Check sheet for the modelled part. Datum: model origin and axes. Units: mm. Give positions to 0.01 mm unless a question says otherwise; leave off trailing zeros. Loops run counter-clockwise (first coordinate to the right, second up) from the corner with the lowest first, then second, coordinate; pieces in that order, holes last. Notation, with made-up numbers: (57, 34.25) - (75, 34.25) arc R19 cw to (75, 63.25) - close; hole circle Ø1 at (65.5, -18). An arc over 180 degrees is marked (long way). Use CSV: the item, a comma, the result in double quotes.
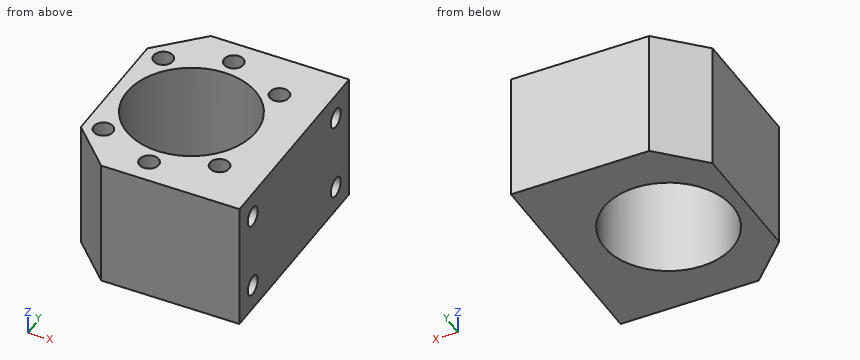
from build123d import *

# Parameters (mm, degrees)
SKETCH1_R           = 20
BOSS_EXTRUDE2_DEPTH = 40
SKETCH8_R           = 3
CUT_EXTRUDE1_DEPTH  = 16
SKETCH9_R           = 3
CUT_EXTRUDE2_DEPTH  = 16


with BuildPart() as part:
    # Sketch1 → Boss-Extrude2 (new body)
    with BuildSketch(Plane.XY):
        Polygon((-24, -20), (-11, -33), (31.93, -33), (31.93, 33), (-11, 33), (-24, 20), align=None)
        Circle(SKETCH1_R, mode=Mode.SUBTRACT)
    extrude(amount=BOSS_EXTRUDE2_DEPTH)

    # Sketch8 → Cut-Extrude1 (cut)
    with BuildSketch(Plane.XY.offset(40)):
        with Locations((0, 25.5)):
            Circle(SKETCH8_R)
        with Locations((18.03122292, 18.03122292)):
            Circle(SKETCH8_R)
        with Locations((18.03122292, -18.03122292)):
            Circle(SKETCH8_R)
        with Locations((0, -25.5)):
            Circle(SKETCH8_R)
        with Locations((-18.03122292, -18.03122292)):
            Circle(SKETCH8_R)
        with Locations((-18.03122292, 18.03122292)):
            Circle(SKETCH8_R)
    extrude(amount=-CUT_EXTRUDE1_DEPTH, mode=Mode.SUBTRACT)

    # Sketch9 → Cut-Extrude2 (cut)
    with BuildSketch(Plane(origin=(31.93, 0, 0), x_dir=(0, 0, -1), z_dir=(1, 0, 0))):
        with Locations((-32, 25)):
            Circle(SKETCH9_R)
        with Locations((-8, 25)):
            Circle(SKETCH9_R)
        with Locations((-8, -25)):
            Circle(SKETCH9_R)
        with Locations((-32, -25)):
            Circle(SKETCH9_R)
    extrude(amount=-CUT_EXTRUDE2_DEPTH, mode=Mode.SUBTRACT)


solid = part.part
1. Sectioned sample at B-B, the plane y = 0. Record the boundary of the cut face in (x, z), and give its area (3 significant figures).
Completed:
outline,"(-24, 0) - (-20, 0) - (-20, 40) - (-24, 40) - close; (20, 0) - (31.93, 0) - (31.93, 40) - (20, 40) - close"
area,"637 mm²"
2. Sectioned sample at C-C, the plane z = 8. Record the boundary of the cut face in (x, y), and give its area (3 significant figures).
Completed:
outline,"(-24, -20) - (-11, -33) - (31.93, -33) - (31.93, -28) - (15.93, -28) - (15.93, -22) - (31.93, -22) - (31.93, 22) - (15.93, 22) - (15.93, 28) - (31.93, 28) - (31.93, 33) - (-11, 33) - (-24, 20) - close; hole circle Ø40 at (0, 0)"
area,"2,070 mm²"
3. Scan lines: line 1 along Y through (x, z) = (21.75, 8); line 2 along Y through (x, z) = (26, 30.5); line 3 along Z through (x, y) = (19.5, 24). Record each from-to range of solid material in increasing order.
Completed:
line 1,"y = -33 to -28, -22 to 22, 28 to 33"
line 2,"y = -33 to -27.6, -22.4 to 22.4, 27.6 to 33"
line 3,"z = 0 to 5.17, 10.83 to 29.17, 34.83 to 40"
4. Sectioned sample at D-D, the plane x = 27.5. Record the boundary of the cut face in (y, z).
Completed:
outline,"(-33, 0) - (33, 0) - (33, 40) - (-33, 40) - close; hole circle Ø6 at (-25, 8); hole circle Ø6 at (-25, 32); hole circle Ø6 at (25, 8); hole circle Ø6 at (25, 32)"
5. Sectioned sample at A-A, the plane x = 0. Record the boundary of the cut face in (y, z), and give its area (3 significant figures).
Completed:
outline,"(-33, 0) - (-20, 0) - (-20, 40) - (-22.5, 40) - (-22.5, 24) - (-28.5, 24) - (-28.5, 40) - (-33, 40) - close; (20, 0) - (33, 0) - (33, 40) - (28.5, 40) - (28.5, 24) - (22.5, 24) - (22.5, 40) - (20, 40) - close"
area,"848 mm²"
6. Go/stop test with flat-tipped pins: pin 1 Ø3.5 at (y, z) = (-25, 32) entering from -X; pin 2 Ø5 at (y, z) = (-25, 8) entering from +X; pin 3 Ø3.5 at (x, y) = (-18.03, 18.03) entering from -Z; pin 4 Ø5 at (y, z) = (25, 32) entering from -X. Record where each tip stops, or that it passes through.
Completed:
pin 1,"stops at x = -20.75"
pin 2,"stops at x = 15.93"
pin 3,"stops at z = 0"
pin 4,"stops at x = -21.5"
